Here's how the part is built. I have some questions about the finished solid (model axes, mm). A direction names the side the tool comes from. Give positions to 0.01 mm unless a question says otherwise; leave off trailing zeros. Loops run counter-clockwise (first coordinate to the right, second up) from the corner with the lowest first, then second, coordinate; pieces in that order, holes last. Notation, with made-up numbers: (28.25, 46.25) - (32.25, 46.25) arc R15 ccw to (32.25, 63.25) - close; hole circle Ø7 at (75.25, -12.5). An arc over 180 degrees is marked (long way). Put each result on its own line as item: value. Start each with the question number.
from build123d import *

# Parameters (mm, degrees)
BOSS_EXTRU_1_DEPTH      = 5
BOSS_EXTRU_1_DEPTH_BACK = 80
ESQUISSE1_W             = 50
ESQUISSE1_H             = 50
BOSS_EXTRU_2_DEPTH      = 50
ENL_V_MAT_EXTRU_2_DEPTH = 133.759180474
COQUE1_START            = -12.344146878
COQUE1_OUTLINE_W        = 40
COQUE1_OUTLINE_H        = 80
COQUE1_DEPTH            = 40
ENL_V_MAT_EXTRU_5_DEPTH = 134.997778874
ENL_V_MAT_EXTRU_6_DEPTH = 10
ENL_V_MAT_EXTRU_7_DEPTH = 134.68023318


# Read off the part's stored shape, not the designer's step: Coque1
with BuildPart() as part:
    # Esquisse1 → Boss.-Extru.1 (new, two sides: drawn at the far end of the back side and taken through both)
    with BuildSketch(Plane.XY.offset(-BOSS_EXTRU_1_DEPTH_BACK)):
        with Locations((25, 7.655853122)):
            Rectangle(ESQUISSE1_W, ESQUISSE1_H)
    extrude(amount=BOSS_EXTRU_1_DEPTH + BOSS_EXTRU_1_DEPTH_BACK)

    # Esquisse2 → Boss.-Extru.2 (add)
    with BuildSketch(Plane(origin=(50, 0, 0), x_dir=(0, 0, -1), z_dir=(1, 0, 0))):
        Polygon((-5, 17.655853122), (45, 17.655853122), (45, -2.344146878), (-5, -2.344146878), (-5, 7.655853122), align=None)
    boss_extru_2 = extrude(amount=BOSS_EXTRU_2_DEPTH)

    # Esquisse5 → Enlèv. mat.-Extru.2 (cut, through all)
    with BuildSketch(Plane.XZ.offset(2.344146878)):
        Polygon((50, -45), (100, 5), (100, -45), align=None)
    enl_v_mat_extru_2 = extrude(amount=-ENL_V_MAT_EXTRU_2_DEPTH, mode=Mode.SUBTRACT)

    # Symétrie2: Boss.-Extru.2, Enlèv. mat.-Extru.2 across plane
    add(boss_extru_2.mirror(Plane.ZY.offset(-25)))
    add(enl_v_mat_extru_2.mirror(Plane.ZY.offset(-25)), mode=Mode.SUBTRACT)

    # Coque1 outline → Coque1 (cut)
    with BuildSketch(Plane(origin=(0, 0, 0), x_dir=(1, 0, 0), z_dir=(0, 1, 0)).offset(COQUE1_START)):
        with Locations((25, 40)):
            Rectangle(COQUE1_OUTLINE_W, COQUE1_OUTLINE_H)
    extrude(amount=COQUE1_DEPTH, mode=Mode.SUBTRACT)

    # Esquisse16 → Enlèv. mat.-Extru.5 (cut, through all)
    with BuildSketch(Plane.XY.offset(3)):
        Polygon((52, 15.655853122), (98, 15.655853122), (98, 7.655853122), (98, -0.344146878), (52, -0.344146878), align=None)
    enl_v_mat_extru_5 = extrude(amount=-ENL_V_MAT_EXTRU_5_DEPTH, mode=Mode.SUBTRACT)

    # Symétrie8: Enlèv. mat.-Extru.5 across plane
    add(enl_v_mat_extru_5.mirror(Plane.ZY.offset(-25)), mode=Mode.SUBTRACT)

    # Esquisse17 → Enlèv. mat.-Extru.6 (cut)
    with BuildSketch(Plane(origin=(0, 0, 3), x_dir=(-1, 0, 0), z_dir=(0, 0, -1))):
        with BuildLine():
            Line((12, 11.720853122), (37, 11.720853122))
            ThreePointArc((37, 11.720853122), (41.065, 7.655853122), (37, 3.590853122))
            Line((37, 3.590853122), (12, 3.590853122))
            ThreePointArc((12, 3.590853122), (7.935, 7.655853122), (12, 11.720853122))
        make_face()
    enl_v_mat_extru_6 = extrude(amount=-ENL_V_MAT_EXTRU_6_DEPTH, mode=Mode.SUBTRACT)

    # Symétrie9: Enlèv. mat.-Extru.6 across plane
    add(enl_v_mat_extru_6.mirror(Plane.ZY.offset(-25)), mode=Mode.SUBTRACT)

    # Esquisse18 → Enlèv. mat.-Extru.7 (cut, through all)
    with BuildSketch(Plane.ZY.offset(2)):
        with BuildLine():
            Line((-65, 11.720853122), (-5, 11.720853122))
            ThreePointArc((-5, 11.720853122), (-0.935, 7.655853122), (-5, 3.590853122))
            Line((-5, 3.590853122), (-65, 3.590853122))
            ThreePointArc((-65, 3.590853122), (-69.065, 7.655853122), (-65, 11.720853122))
        make_face()
    extrude(amount=-ENL_V_MAT_EXTRU_7_DEPTH, mode=Mode.SUBTRACT)


solid = part.part
1) Thinking about a two-plate mould opening in Z: for faces 6 (the flat face through (48, 11.721, -35)), 7 (the flat face through (-25, 13, 3)), 8 (the flat face through (0, 2, -48)), which applies, pulls with the +Z half, pulls with the -Z half, needs draft (parallel to the pull), parting line crosses it, or undercut?
2) I'm going to push flat-ended pins straight in: P1, Ø2, axis at x = 72.5, z = 4, coming from the +Y side; P2, Ø1.5, axis at y = 18.5, z = -60.5, coming from the -X side; P3, Ø5, axis at x = -31.5, y = 11, coming from the -Z side; P4, Ø10, axis at x = 77, y = -3, coming from the +Z side. Where does each tip first touch, or does it pass through?
3) Which directions (+Z, -Z, +X, -X, +Y, -Y) give clear straight access to the entire face, cutting with the end or side of a thin tool? Please do faces 1 (the flat face through (-2, 2, -20)), 2 (the flat face through (52, 2, -20)), 3 (the flat face through (25, 7, 0)), 4 (the cylindrical face through (-41.064, 7.745, 3.986)), 5 (the flat face through (69, 17.656, -14)).
4) Suppose I cut it at C-C on y = -7. Please give me the cut outline in (x, z), plus the area to 3 significant figures.
5) I need wall thicknesses on line 1 (X direction, y = -3.5, z = -24); line 2 (Y direction, x = 42, z = -33); line 3 (Y direction, x = -19, z = -6.5). Which ranges of each line are inside material? Lowest first, please.
6) Suppose I cut it at D-D on z = -71.5. Please give me the cut outline in (x, y), plus the area to 3 significant figures.
7) Suppose I cut it at B-B on x = -18. Please give me the cut outline in (y, z), plus the area to 3 significant figures.
Ans:
1. face 6: undercut
1. face 7: pulls with the -Z half
1. face 8: needs draft
2. P1: stops at y = 17.66
2. P2: stops at x = 0
2. P3: stops at z = 3
2. P4: stops at z = 5
3. face 1: -Z, -X
3. face 2: -Z, +X
3. face 3: -Z
3. face 4: +Z, -Z
3. face 5: +Z, -Z, +X, +Y
4. outline: (0, -80) - (5, -80) - (5, 0) - (45, 0) - (45, -80) - (50, -80) - (50, 5) - (0, 5) - close
4. area: 1,050 mm²
5. line 1: x = 0 to 5, 45 to 50
5. line 2: y = -17.34 to -12.34, 27.66 to 32.66
5. line 3: y = -2.34 to -0.34, 15.66 to 17.66
6. outline: (0, -17.34) - (50, -17.34) - (50, 32.66) - (0, 32.66) - close; hole (5, -12.34) - (45, -12.34) - (45, 27.66) - (5, 27.66) - close
6. area: 900 mm²
7. outline: (-2.34, -27) - (-0.34, -27) - (-0.34, 3) - (3.59, 3) - (3.59, 5) - (-2.34, 5) - close; (11.72, 3) - (15.66, 3) - (15.66, -27) - (17.66, -27) - (17.66, 5) - (11.72, 5) - close
7. area: 144 mm²
